```python
from build123d import *

# Parameters (mm, degrees)
SKETCH1_W           = 77
SKETCH1_H           = 50
BOSS_EXTRUDE1_DEPTH = 2
SKETCH2_W           = 77
SKETCH2_H           = 2
BOSS_EXTRUDE2_DEPTH = 67.75
CUT_EXTRUDE1_DEPTH  = 81.835094483
BOSS_EXTRUDE3_DEPTH = 2
FILLET1_R           = 1


with BuildPart() as part:
    # Sketch1 → Boss-Extrude1 (new body)
    with BuildSketch(Plane(origin=(0, 0, 0), x_dir=(1, 0, 0), z_dir=(0, 1, 0))):
        Rectangle(SKETCH1_W, SKETCH1_H)
    extrude(amount=BOSS_EXTRUDE1_DEPTH)

    # Sketch2 → Boss-Extrude2 (add)
    with BuildSketch(Plane.XZ):
        with Locations((0, 26)):
            Rectangle(SKETCH2_W, SKETCH2_H)
    extrude(amount=-BOSS_EXTRUDE2_DEPTH)

    # Sketch3 → Cut-Extrude1 (cut, through all)
    with BuildSketch(Plane(origin=(0, 2, 0), x_dir=(1, 0, 0), z_dir=(0, 1, 0))):
        with BuildLine():
            Line((2, 25), (2, -15))
            ThreePointArc((2, -15), (0, -17), (-2, -15))
            Line((-2, -15), (-2, 25))
            Line((-2, 25), (2, 25))
        make_face()
    extrude(amount=-CUT_EXTRUDE1_DEPTH, mode=Mode.SUBTRACT)

    # Sketch4 → Boss-Extrude3 (add)
    with BuildSketch(Plane(origin=(0, 2, 0), x_dir=(1, 0, 0), z_dir=(0, 1, 0))):
        Polygon((-38.5, 25), (-40, 23.212369611), (-38.5, 22.346344207), align=None)
        Polygon((40, 23.212369611), (38.5, 22.346344207), (38.5, 25), align=None)
    extrude(amount=-BOSS_EXTRUDE3_DEPTH)

    # Fillet1
    fillet1_edges = [part.edges().sort_by_distance(p)[0] for p in [
        (-40, 1, -23.212369611),
        (40, 1, -23.212369611),
        (-38.5, 1, -25),
        (38.5, 1, -25),
    ]]
    fillet(fillet1_edges, radius=FILLET1_R)


solid = part.part
```
The listing builds one solid part. Answer for the finished solid, in the listing's coordinates (mm). A direction names the side the tool comes from. Give positions to 0.01 mm unless a question says otherwise; leave off trailing zeros. Write each loop counter-clockwise with the first axis right and the second up, starting at its lowest first coordinate (ties: lowest second). Pieces come first, ordered by that corner, then holes. Notation, with made-up numbers: (43, 64) -> (75, 64) arc R20 cw to (75, 100) -> close; hole circle Ø3 at (-9, 50.25). An arc over 180 degrees is marked (long way). Use one line per item in the form item = value.
1) Straight lines are drawn through the part: probe 1 along Y at (x, z) = (6.5, -19.5); probe 2 along Z at (x, y) = (12.5, 44.5). For each, find the intervals that lie inside material, in ascending order.
Result:
probe_1 = 0 to 2
probe_2 = 25 to 27
2) Section A-A on z = 9 is taken. Write down the section's boundary in (x, y), plus the area to 3 significant figures.
Result:
outline = (-38.5, 0) -> (-2, 0) -> (-2, 2) -> (-38.5, 2) -> close; (2, 0) -> (38.5, 0) -> (38.5, 2) -> (2, 2) -> close
area = 146 mm²
3) Section C-C on x = 0 is taken. Write down the section's boundary in (y, z), plus the area to 4 significant figures.
Result:
outline = (0, 17) -> (2, 17) -> (2, 25) -> (67.75, 25) -> (67.75, 27) -> (0, 27) -> close
area = 151.5 mm²
4) A tool of negligible diameter and unlimited length cuts with its end or side. For faces 1 (the flat face through (-1, 33, 27)), 2 (the flat face through (2, 1, -5)), 3 (the flat face through (-38.5, 19, 26)), 4 (the flat face through (-1, 34, 25)), from which of +Z, -Z, +X, -X, +Y, -Y can it reach the whole face along a straight path? Write none if from no direction.
Result:
face_1 = +Z, +X, -X, +Y, -Y
face_2 = -Z, +Y, -Y
face_3 = +Z, -X, +Y, -Y
face_4 = -Z, +X, -X, +Y
5) Each of these flat-tipped pins is pushed along its axis until it touches: P1, Ø15, axis at x = 8, z = 2.5, coming from the +Y side; P2, Ø2, axis at y = 1, z = -7, coming from the +X side; P3, Ø0.6, axis at y = 1, z = -4, coming from the -X side. Where does it stop, or does it pass through?
Result:
P1 = 2
P2 = 38.5
P3 = -38.5
6) For a pull along X with two mould halves and no side action, classify faces 5 (the flat face through (38.5, 19, 26)), 6 (the flat face through (-1, 67.75, 26)), 7 (the flat face through (-2, 1, -5)) as +X half, -X half, draft (parallel to the pull), parting line (faces both ways), or undercut.
Result:
face_5 = +X half
face_6 = draft
face_7 = undercut
7) Section B-B on x = 26.5 is taken. Write down the section's boundary in (y, z).
Result:
outline = (0, -25) -> (2, -25) -> (2, 25) -> (67.75, 25) -> (67.75, 27) -> (0, 27) -> close
8) Section D-D on y = 63 is taken. Write down the section's boundary in (x, z), plus the area to 3 significant figures.
Result:
outline = (-38.5, 25) -> (38.5, 25) -> (38.5, 27) -> (-38.5, 27) -> close
area = 154 mm²
